For this review, use the dimensioned drawing (mm, ordinates from the lowest corner) and the shaded views. Round coordinates to 2 decimals unless told otherwise and drop trailing zeros. Write each loop counter-clockwise with the first axis right and the second up, starting at its lowest first coordinate (ties: lowest second). Pieces come first, ordered by that corner, then holes. Notation, with made-up numbers: M 15.25,62.25 L 42.25,62.25 A25 ccw 42.25,88.25 Z; hole C -21,-24.5 d8. An arc over 180 degrees is marked long. Use one line per item in the form item = value. Start each with the question number.
Item 1: Add section C-C (y = 3.2). State the section outline as (x, z) points.
Item 2: Add section B-B (z = 25). State the section outline as (x, y) points, and give its area (3 significant figures).
Item 3: Add section A-A (x = 131). State the section outline as (y, z) points.
Item 4: For line 1 (Z direction, x = 20, y = 1.45); line 2 (Z direction, x = 59, y = 2.75); line 3 (X direction, y = 4.45, z = 13), list the stretches that pass through material, from the lowest coordinate up. Write a range as [from, to].
Item 5: Add section D-D (x = 76). State the section outline as (y, z) points.
Item 6: For P1, Ø1.7, axis at x = 20, z = 25, coming from the +Y side; P2, Ø2.5, axis at x = 94.5, y = 2, coming from the -Z side; P3, Ø1.5, axis at y = 1.5, z = 44, coming from the +X side; P4, Ø2.5, axis at x = 65, y = 3.5, coming from the +Z side, all flat-tipped, find the tip position at first contact; note any pin that passes through.
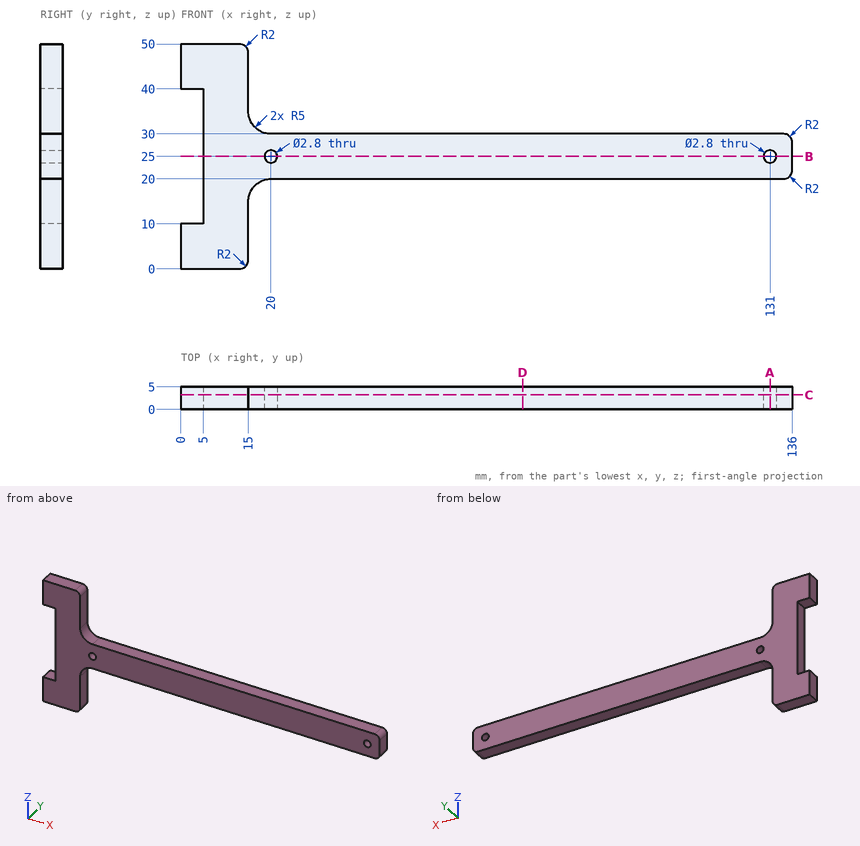
Calculated:
q1.outline = M 0,0 L 13,0 A2 ccw 15,2 L 15,15 A5 cw 20,20 L 134,20 A2 ccw 136,22 L 136,28 A2 ccw 134,30 L 20,30 A5 cw 15,35 L 15,48 A2 ccw 13,50 L 0,50 L 0,40 L 5,40 L 5,10 L 0,10 Z; hole C 20,25 d2.8; hole C 131,25 d2.8
q2.outline = M 5,0 L 18.6,0 L 18.6,5 L 5,5 Z; M 21.4,0 L 129.6,0 L 129.6,5 L 21.4,5 Z; M 132.4,0 L 136,0 L 136,5 L 132.4,5 Z
q2.area = 627 mm^2
q3.outline = M 0,20 L 5,20 L 5,23.6 L 0,23.6 Z; M 0,26.4 L 5,26.4 L 5,30 L 0,30 Z
q4.line_1 = [20, 23.6], [26.4, 30]
q4.line_2 = [20, 30]
q4.line_3 = [5, 15]
q5.outline = M 0,20 L 5,20 L 5,30 L 0,30 Z
q6.P1 = through
q6.P2 = 20
q6.P3 = 15
q6.P4 = 30
